Job drawing, mm, ordinate dimensions from the low corner. One solid piece. A direction names the side the tool comes from. Give positions to 0.01 mm unless a question says otherwise; leave off trailing zeros. Write each loop counter-clockwise with the first axis right and the second up, starting at its lowest first coordinate (ties: lowest second). Pieces come first, ordered by that corner, then holes. Notation, with made-up numbers: M 3,-31.5 L 12,-31.5 A15 cw 12,-5.5 Z; hole C -19,89.25 d4. An arc over 180 degrees is marked long. Use a Markdown table: item, result.
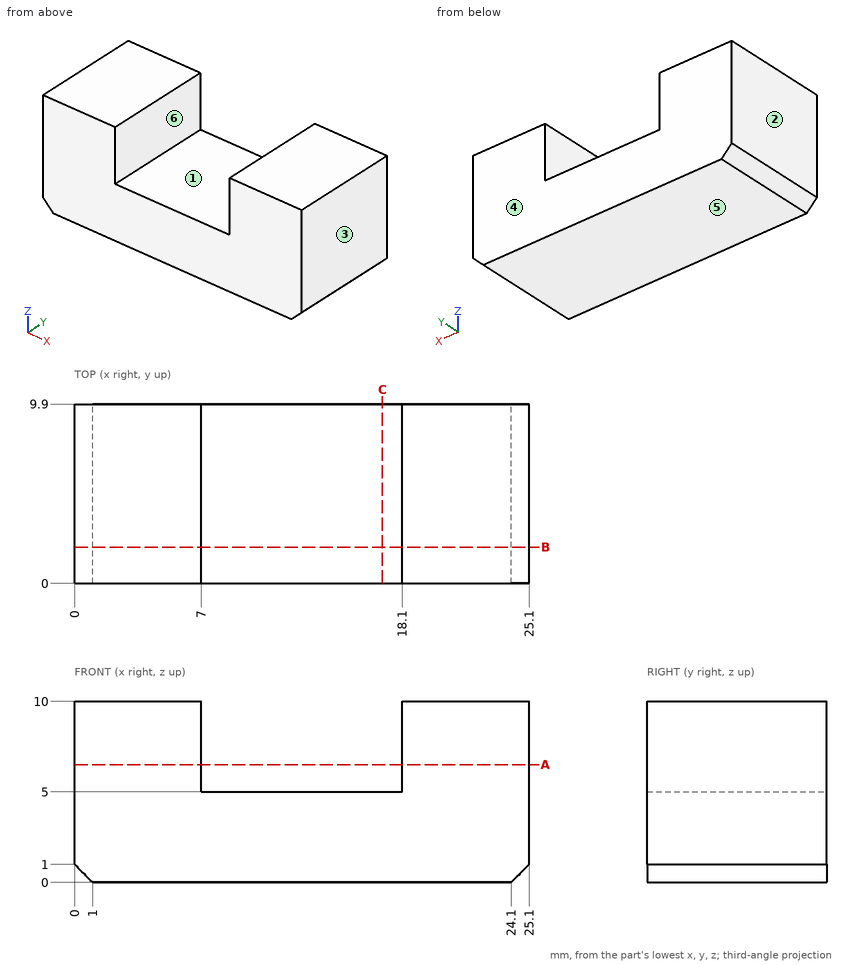
1. Two-plate mould, pull along X, no slides. Class the marked faces 1, 2, 3 and 4: released by +X, released by -X, zero draft, split by the parting line, or undercut.
Findings below:
| item | result |
|---|---|
| face 1 | undercut |
| face 2 | released by -X |
| face 3 | released by +X |
| face 4 | zero draft |
2. Cut at C-C, the plane x = 17. Give the cut face in (y, z), then the cut area to 3 significant figures.
Findings below:
| item | result |
|---|---|
| outline | M 0,0 L 9.9,0 L 9.9,5 L 0,5 Z |
| area | 49.5 mm2 |
3. Cut at A-A, the plane z = 6.5. Give the cut face in (x, y).
Findings below:
| item | result |
|---|---|
| outline | M 0,0 L 7,0 L 7,9.9 L 0,9.9 Z; M 18.1,0 L 25.1,0 L 25.1,9.9 L 18.1,9.9 Z |
4. Drop a flat-ended pin along its axis: P1, Ø5, axis at x = 15.5, y = 5, coming from the +Z side. Give the stop position or say it passes through.
Findings below:
| item | result |
|---|---|
| P1 | z = 5 |
5. Drill centre lines: L1, parallel to X at y = 5.5, z = 5.5; L2, parallel to Z at x = 16.25, y = 0.75; L3, parallel to X at y = 5.25, z = 0.75. Where is each one in solid material? Low to high.
Findings below:
| item | result |
|---|---|
| L1 | 0 to 7, 18.1 to 25.1 |
| L2 | 0 to 5 |
| L3 | 0.25 to 24.85 |
6. Tool access for the marked faces 5 and 6: list every direction of +Z, -Z, +X, -X, +Y, -Y with a clear straight run to the whole face (end or side of a thin tool).
Findings below:
| item | result |
|---|---|
| face 5 | -Z, +X, -X, +Y, -Y |
| face 6 | +Z, +Y, -Y |
7. Cut at B-B, the plane y = 2. Give the cut face in (x, z), then the cut area to 4 significant figures.
Findings below:
| item | result |
|---|---|
| outline | M 0,1 L 1,0 L 24.1,0 L 25.1,1 L 25.1,10 L 18.1,10 L 18.1,5 L 7,5 L 7,10 L 0,10 Z |
| area | 194.5 mm2 |
